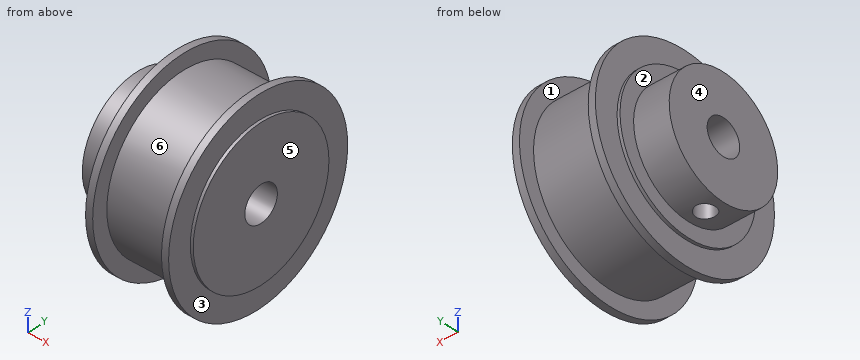
```python
from build123d import *

# Parameters (mm, degrees)
CROQUIS1_R                = 10
SALIENTE_EXTRUIR1_DEPTH   = 6
CROQUIS2_R                = 12.5
SALIENTE_EXTRUIR2_DEPTH   = 0.5
CROQUIS3_R                = 16.5
SALIENTE_EXTRUIR3_DEPTH   = 1.2
CROQUIS4_R                = 13.9
SALIENTE_EXTRUIR4_DEPTH   = 11.6
CROQUIS5_R                = 16.5
SALIENTE_EXTRUIR5_DEPTH   = 1.2
CROQUIS6_R                = 12.5
SALIENTE_EXTRUIR6_DEPTH   = 0.5
CROQUIS7_R                = 3
CORTAR_EXTRUIR1_DEPTH     = 32.392674305
TALADRO_ROSCADO_M41_D     = 3.3
TALADRO_ROSCADO_M41_DEPTH = 11.5
TALADRO_ROSCADO_M41_TIP   = 0.991420021


with BuildPart() as part:
    # Croquis1 → Saliente-Extruir1 (new body)
    with BuildSketch(Plane(origin=(0, 0, 0), x_dir=(0, 0, -1), z_dir=(1, 0, 0))):
        Circle(CROQUIS1_R)
    extrude(amount=SALIENTE_EXTRUIR1_DEPTH)

    # Croquis2 → Saliente-Extruir2 (add)
    with BuildSketch(Plane(origin=(6, 0, 0), x_dir=(0, 0, -1), z_dir=(1, 0, 0))):
        Circle(CROQUIS2_R)
    extrude(amount=SALIENTE_EXTRUIR2_DEPTH)

    # Croquis3 → Saliente-Extruir3 (add)
    with BuildSketch(Plane(origin=(6.5, 0, 0), x_dir=(0, 0, -1), z_dir=(1, 0, 0))):
        Circle(CROQUIS3_R)
    extrude(amount=SALIENTE_EXTRUIR3_DEPTH)

    # Croquis4 → Saliente-Extruir4 (add)
    with BuildSketch(Plane(origin=(7.7, 0, 0), x_dir=(0, 0, -1), z_dir=(1, 0, 0))):
        Circle(CROQUIS4_R)
    extrude(amount=SALIENTE_EXTRUIR4_DEPTH)

    # Croquis5 → Saliente-Extruir5 (add)
    with BuildSketch(Plane(origin=(19.3, 0, 0), x_dir=(0, 0, -1), z_dir=(1, 0, 0))):
        Circle(CROQUIS5_R)
    extrude(amount=SALIENTE_EXTRUIR5_DEPTH)

    # Croquis6 → Saliente-Extruir6 (add)
    with BuildSketch(Plane(origin=(20.5, 0, 0), x_dir=(0, 0, -1), z_dir=(1, 0, 0))):
        Circle(CROQUIS6_R)
    extrude(amount=SALIENTE_EXTRUIR6_DEPTH)

    # Croquis7 → Cortar-Extruir1 (cut, through all)
    with BuildSketch(Plane.ZY):
        Circle(CROQUIS7_R)
    extrude(amount=-CORTAR_EXTRUIR1_DEPTH, mode=Mode.SUBTRACT)

    # Taladro roscado M41
    with Locations(Plane(origin=(0, 0, -10), x_dir=(-1, 0, 0), z_dir=(0, 0, -1))):
        with Locations((-3, 0)):
            Hole(TALADRO_ROSCADO_M41_D / 2, depth=TALADRO_ROSCADO_M41_DEPTH)
            with Locations((0, 0, -(TALADRO_ROSCADO_M41_DEPTH + TALADRO_ROSCADO_M41_TIP / 2))):  # 118° drill point
                Cone(0, TALADRO_ROSCADO_M41_D / 2, TALADRO_ROSCADO_M41_TIP, mode=Mode.SUBTRACT)


solid = part.part
```
Read the model definition and answer for the solid it produces. Units are mm, in the model's axes. Face numbers are marked on the shaded views. A direction names the side the tool comes from. Round coordinates to 2 decimals unless told otherwise and drop trailing zeros. Write each loop counter-clockwise with the first axis right and the second up, starting at its lowest first coordinate (ties: lowest second). Pieces come first, ordered by that corner, then holes. Notation, with made-up numbers: M 15.25,-10.5 L 54.25,-10.5 A9 ccw 54.25,-1.5 Z; hole C 37.25,31 d11. An arc over 180 degrees is marked long. One line per item, written item: value.
Q1. Flat-ended cylindrical pins translate along their axes: pin 1 Ø8 at (x, z) = (18.5, 7) entering from -Y; pin 2 Ø2.5 at (x, y) = (3, 0) entering from +Z; pin 3 Ø8 at (x, y) = (6.5, -12) entering from +Z. Find the tip coordinate at first contact, or state that the pin passes through.
Data:
pin 1: y = -16.21
pin 2: z = 10
pin 3: z = 14.43
Q2. Which of the six approach directions +Z, -Z, +X, -X, +Y, -Y give full straight-line access (tool end or side, diameter ignored) to the marked faces 1, 2 and 3?
Data:
face 1: none
face 2: -X
face 3: +X
Q3. For a pull along X with two mould halves and no side action, classify the marked faces 4, 5 and 6 as +X half, -X half, draft (parallel to the pull), parting line (faces both ways), or undercut.
Data:
face 4: -X half
face 5: +X half
face 6: undercut
Q4. Find section B-B on y = 0. Count the separate pieces of the cut face and the enclosed holes in it, plus the area to 3 significant figures.
Data:
separate pieces: 3
enclosed holes: 0
area: 398 mm2
Q5. Straight lines are drawn through the part: line 1 (X direction, y = 6, z = -15); line 2 (X direction, y = 0, z = -8.25); line 3 (Y direction, x = 11, z = 0). For each, find the intervals that lie inside material, in ascending order. Write a range as [from, to].
Data:
line 1: [6.5, 7.7], [19.3, 20.5]
line 2: [0, 1.35], [4.65, 21]
line 3: [-13.9, -3], [3, 13.9]
Q6. Find section C-C on x = 5.25. Write down the section's boundary in (y, z), plus the area to 3 significant figures.
Data:
outline: C 0,0 d20; hole C 0,0 d6
area: 286 mm2
Q7. Find section A-A on z = 0. Write down the section's boundary in (x, y), plus the area to 3 significant figures.
Data:
outline: M 0,-10 L 6,-10 L 6,-12.5 L 6.5,-12.5 L 6.5,-16.5 L 7.7,-16.5 L 7.7,-13.9 L 19.3,-13.9 L 19.3,-16.5 L 20.5,-16.5 L 20.5,-12.5 L 21,-12.5 L 21,-3 L 0,-3 Z; M 0,3 L 21,3 L 21,12.5 L 20.5,12.5 L 20.5,16.5 L 19.3,16.5 L 19.3,13.9 L 7.7,13.9 L 7.7,16.5 L 6.5,16.5 L 6.5,12.5 L 6,12.5 L 6,10 L 0,10 Z
area: 421 mm2
Q8. Find section D-D on z = -7.5. Write down the section's boundary in (x, y).
Data:
outline: M 0,-6.61 L 6,-6.61 L 6,-10 L 6.5,-10 L 6.5,-14.7 L 7.7,-14.7 L 7.7,-11.7 L 19.3,-11.7 L 19.3,-14.7 L 20.5,-14.7 L 20.5,-10 L 21,-10 L 21,10 L 20.5,10 L 20.5,14.7 L 19.3,14.7 L 19.3,11.7 L 7.7,11.7 L 7.7,14.7 L 6.5,14.7 L 6.5,10 L 6,10 L 6,6.61 L 0,6.61 Z; hole C 3,0 d3.3
